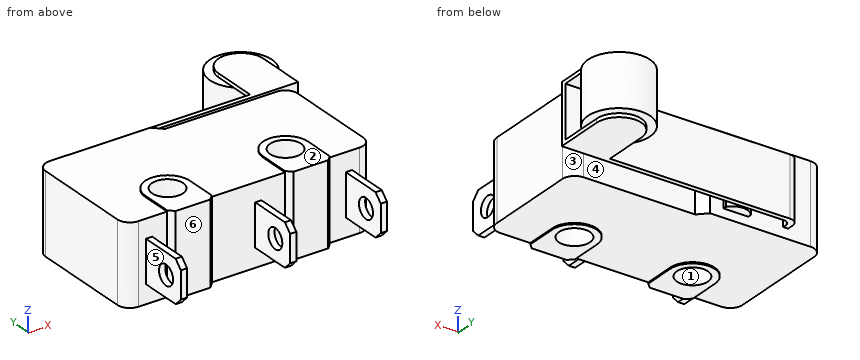
Autodesk Inventor part; units mm, degrees
ref_plane "YZ Plane" through (0, 0, 0) normal (1, 0, 0) x (0, 1, 0)
ref_plane "XZ Plane" through (0, 0, 0) normal (0, 1, 0) x (-1, 0, 0)
ref_plane "XY Plane" through (0, 0, 0) normal (0, 0, 1) x (1, 0, 0)
sketch "Эскиз2" plane through (0, 0, 0) normal (0, 0, 1) x (1, 0, 0)
  line L0 (1, 0) -> (18.8, 0)
  line L1 (19.8, 1) -> (19.8, 8.5)
  line L2 (18.8, 9.5) -> (9.8, 9.5)
  line L3 (9.8, 9.5) -> (9.1, 10.2)
  line L4 (9.1, 10.2) -> (1, 10.2)
  line L5 (0, 9.2) -> (0, 1)
  arc A0 (1, 10.2) -> (0, 9.2) centre (1, 9.2) ccw
  arc A1 (0, 1) -> (1, 0) centre (1, 1) ccw
  arc A2 (18.8, 0) -> (19.8, 1) centre (18.8, 1) ccw
  arc A3 (19.8, 8.5) -> (18.8, 9.5) centre (18.8, 8.5) ccw
  point P0 (0, 0)
  point P1 (19.8, 0)
  point P2 (19.8, 9.5)
  dimension "d42" = 19.8
  dimension "d43" = 9.5
  dimension "d44" = 10
  dimension "d45" = 135
  dimension "d46" = 10.2
  dimension "d47" = 1
extrude "Выдавливание1" add sketch "Эскиз2" along normal mid plane 6.4
sketch "Эскиз3" plane through (0, 0, 0) normal (0, 0, 1) x (1, 0, 0)
  line L0 (1, 0) -> (18.8, 0)
  line L1 (1.6, 0) -> (2.1, 0)
  line L2 (2.1, 0) -> (2.1, -4)
  line L3 (2.1, -4) -> (1.6, -4)
  line L4 (1.6, -4) -> (1.6, 0)
  line L5 (10.4, 0) -> (10.9, 0)
  line L6 (10.9, 0) -> (10.9, -4)
  line L7 (10.9, -4) -> (10.4, -4)
  line L8 (10.4, -4) -> (10.4, 0)
  line L9 (17.7, 0) -> (18.2, 0)
  line L10 (18.2, 0) -> (18.2, -4)
  line L11 (18.2, -4) -> (17.7, -4)
  line L12 (17.7, -4) -> (17.7, 0)
  line L13 (0, 9.2) -> (0, 1)
  point P0 (0, 0)
  point P1 (1.85, -4)
  point P2 (17.95, -4)
  point P3 (10.65, -4)
  dimension "d51" = 0.5
  dimension "d52" = 8.8
  dimension "d53" = 7.3
  dimension "d54" = 4
  dimension "d55" = 1.85
extrude "Выдавливание2" add sketch "Эскиз3" along normal mid plane 3.4
sketch "Эскиз4" plane through (0, 0, 0) normal (0, 0, 1) x (1, 0, 0)
  arc A0 (6.9, 2.5) -> (3.3, 2.5) centre (5.1, 2.5) ccw
  line L0 (3.3, 2.5) -> (3.3, 0)
  line L1 (18.8, 0) -> (1, 0)
  line L2 (3.3, 0) -> (3.7, -0.4)
  line L3 (3.7, -0.4) -> (6.5, -0.4)
  line L4 (6.5, -0.4) -> (6.9, 0)
  line L5 (6.9, 0) -> (6.9, 2.5)
  line L6 (12.8, 0) -> (13.2, -0.4)
  line L7 (13.2, -0.4) -> (16, -0.4)
  line L8 (16, -0.4) -> (16.4, 0)
  line L9 (16.4, 0) -> (16.4, 2.5)
  line L10 (12.8, 0) -> (12.8, 2.5)
  arc A1 (16.4, 2.5) -> (12.8, 2.5) centre (14.6, 2.5) ccw
  line L11 (0, 1) -> (0, 9.2)
  point P0 (0, 0)
  dimension "d58" = 0.4
  dimension "d59" = 2.5
  dimension "d60" = 1.8
  dimension "d61" = 135
  dimension "d62" = 9.5
  dimension "d63" = 5.1
extrude "Выдавливание3" add sketch "Эскиз4" along normal mid plane 6.6
sketch "Эскиз6" plane through (0, 0, 3.3) normal (0, 0, 1) x (1, 0, 0)
  arc A0 (6.9, 2.5) -> (3.3, 2.5) centre (5.1, 2.5) ccw
  arc A1 (16.4, 2.5) -> (12.8, 2.5) centre (14.6, 2.5) ccw
  point P0 (0, 0)
hole "Отверстие1" at (5.1, 2.5, 3.3) at (14.6, 2.5, 3.3) direction (0, 0, -1) diameter 2.5 end through all
sketch "Эскиз7" plane through (0, 0, 0) normal (0, 0, 1) x (1, 0, 0)
  line L0 (1, 10.2) -> (9.1, 10.2)
  line L1 (2.8, 10.2) -> (2.8, 10.7)
  line L2 (3.5, 11.4) -> (18, 11.4)
  line L3 (18, 11.4) -> (18, 15)
  line L4 (21.6, 15) -> (21.6, 11)
  line L5 (21.6, 11) -> (3.7, 11)
  line L6 (3.2, 10.5) -> (3.2, 10.2)
  arc A0 (21.6, 15) -> (18, 15) centre (19.8, 15) ccw
  line L7 (0, 9.2) -> (0, 1)
  arc A1 (3.7, 11) -> (3.2, 10.5) centre (3.7, 10.5) ccw
  arc A2 (3.5, 11.4) -> (2.8, 10.7) centre (3.5, 10.7) ccw
  point P0 (0, 0)
  point P1 (2.8, 11.4)
  point P2 (3.2, 11)
  dimension "d73" = 0.4
  dimension "d74" = 2.8
  dimension "d75" = 17
  dimension "d76" = 1.8
  dimension "d77" = 0.4
  dimension "d78" = 0.8
  dimension "d79" = 4
  dimension "d82" = 0.5
  dimension "d83" = 0.7
extrude "Выдавливание4" add sketch "Эскиз7" along normal mid plane 4.8
sketch "Эскиз8" plane through (0, 0, 0) normal (0, 0, 1) x (1, 0, 0)
  line L0 (3.5, 11.4) -> (18, 11.4)
  line L1 (9.8542, 11.4) -> (26.7526, 11.4)
  line L2 (26.7526, 11.4) -> (26.7526, 19.641)
  line L3 (26.7526, 19.641) -> (9.8542, 19.641)
  line L4 (9.8542, 19.641) -> (9.8542, 11.4)
  point P0 (0, 0)
  point P1 (19.8, 15)
extrude "Выдавливание5" cut sketch "Эскиз8" along normal mid plane 4.2
sketch "Эскиз9" plane through (0, 0, 0) normal (0, 0, 1) x (1, 0, 0)
  arc A0 (21.6, 15) -> (18, 15) centre (19.8, 15) ccw
  circle A1 centre (19.8, 15) radius 2.5
  point P0 (0, 0)
  dimension "d87" = 5
extrude "Выдавливание6" add sketch "Эскиз9" along normal mid plane 4.2
sketch "Эскиз10" plane through (1.6, -4, 1.7) normal (-1, 0, 0) x (0, 0, 1)
  circle A0 centre (-1.7, 1.7) radius 0.8
  line L0 (-3.4, 0) -> (0, 0)
  point P0 (-1.7, 4)
  dimension "d90" = 1.6
  dimension "d91" = 1.7
extrude "Выдавливание7" cut sketch "Эскиз10" against normal through all
chamfer "Фаска1" distance 0.6 angle 45 6 edges at (1.85, -4, -1.7) (10.65, -4, -1.7) (17.95, -4, -1.7) (10.65, -4, 1.7) (1.85, -4, 1.7) (17.95, -4, 1.7)
sketch "Эскиз11" plane through (0, 0, 0) normal (0, 0, 1) x (1, 0, 0)
  arc A0 (8, 10.4633) -> (6, 10.4633) centre (7, 9.8) ccw
  line L0 (6, 10.4633) -> (6, 10.2)
  line L1 (6, 10.2) -> (8, 10.2)
  line L2 (9.1, 10.2) -> (1, 10.2)
  line L3 (8, 10.4633) -> (8, 10.2)
  line L4 (3.7, 11) -> (21.6, 11)
  line L5 (0, 9.2) -> (0, 1)
  point P0 (0, 0)
  dimension "d97" = 1.2
  dimension "d98" = 2
  dimension "d99" = 6
extrude "Выдавливание8" add sketch "Эскиз11" along normal mid plane 5
properties part number "MSW-13" material "Пластик АБС"
Here's how the part is built. I have some questions about the finished solid (model axes, mm). Face numbers are marked on the shaded views. A direction names the side the tool comes from. Coordinates: 2 decimals unless noted, no trailing zeros. Loops run counter-clockwise (first coordinate to the right, second up) from the corner with the lowest first, then second, coordinate; pieces in that order, holes last. Notation, with made-up numbers: (-22.5, -32) - (-13.5, -32) arc R12 cw to (-13.5, -12) - close; hole circle Ø7 at (-22, 21). An arc over 180 degrees is marked (long way). Return JSON: item names as keys, results as strings. Group by question number.
Item 1: Will these pins go through, and if not, where does the flat tip stop? P1, Ø5.5, axis at x = 12, y = 14.5, coming from the +Z side; P2, Ø2, axis at x = 14.5, z = 1, coming from the -Y side; P3, Ø2, axis at x = 9, z = 0, coming from the +Y side; P4, Ø1.5, axis at x = 19.5, y = 3.5, coming from the -Z side.
Item 2: If we section it at D-D on x = 16.75: Write out the boundary of the cut face in (y, z), and give its area (3 significant figures).
Item 3: If we section it at A-A on x = 5.1: Write out the boundary of the cut face in (y, z).
Item 4: We'd pull the mould along X, two halves only. Please class the marked faces 1, 2 and 3: +X half, -X half, draft (parallel to the pull), parting line (faces both ways), or undercut.
Item 5: If we section it at B-B on y = -1: Write out the boundary of the cut face in (x, z).
Item 6: I need wall thicknesses on line 1 (Y direction, x = 14.6, z = 1.25); line 2 (Y direction, x = 1.85, z = 0); line 3 (Y direction, x = 5, z = 2.75). Which ranges of each line are inside material? Lowest first, please. Write a range as from..to.
Item 7: If we section it at C-C on z = 0: State how many separate pieces and enclosed holes the cut face has, and give its area (3 significant figures).
Item 8: On a 3-axis mill with a long thin cutter (end or side, diameter ignored), from which of +Z, -Z, +X, -X, +Y, -Y can I reach the whole of each face in a straight line? I mean the marked faces 4, 5 and 6. Say none if no direction works.
Calculated:
{
 "1": {"P1": "passes through", "P2": "stops at y = -0.4", "P3": "stops at y = 11.4", "P4": "stops at z = -3.2"},
 "2": {"outline": "(0, -3.2) - (9.5, -3.2) - (9.5, 3.2) - (0, 3.2) - close; (11, -2.4) - (11.4, -2.4) - (11.4, 2.4) - (11, 2.4) - close", "area": "62.7 mm^2"},
 "3": {"outline": "(-0.4, -3.3) - (1.25, -3.3) - (1.25, 3.3) - (-0.4, 3.3) - close; (3.75, -3.3) - (4.3, -3.3) - (4.3, -3.2) - (10.2, -3.2) - (10.2, 3.2) - (4.3, 3.2) - (4.3, 3.3) - (3.75, 3.3) - close; (11, -2.4) - (11.4, -2.4) - (11.4, 2.4) - (11, 2.4) - close"},
 "4": {"face 1": "undercut", "face 2": "draft", "face 3": "+X half"},
 "5": {"outline": "(1.6, -1.7) - (2.1, -1.7) - (2.1, 1.7) - (1.6, 1.7) - close; (10.4, -1.7) - (10.9, -1.7) - (10.9, 1.7) - (10.4, 1.7) - close; (17.7, -1.7) - (18.2, -1.7) - (18.2, 1.7) - (17.7, 1.7) - close"},
 "6": {"line 1": "y = -0.4..1.25, 3.75..9.5, 11..11.4", "line 2": "y = -4..-3.1, -1.5..10.2", "line 3": "y = -0.4..1.25, 3.75..10.2"},
 "7": {"separate pieces": "5", "enclosed holes": "2", "area": "219 mm^2"},
 "8": {"face 4": "+Z, -Z, +X", "face 5": "+Z, -Z, -X, -Y", "face 6": "+Z, -Z, -Y"}
}
